Source: CAD feature listing. Evaluate the final solid. Frame: model axes, mm. Face numbers are marked on the shaded views. A direction names the side the tool comes from. Give positions to 0.01 mm unless a question says otherwise; leave off trailing zeros. Loops run counter-clockwise (first coordinate to the right, second up) from the corner with the lowest first, then second, coordinate; pieces in that order, holes last. Notation, with made-up numbers: (10, 51) -> (66, 51) arc R24 ccw to (66, 69) -> close; hole circle Ø4 at (16.25, -12). An arc over 180 degrees is marked (long way). Put each result on its own line as item: value.
```python
from build123d import *

# Parameters (mm, degrees)
BOSS_EXTRUDE1_DEPTH       = 8
CUT_EXTRUDE1_DEPTH        = 46
M2X0_4_TAPPED_HOLE1_D     = 1.6
M2X0_4_TAPPED_HOLE1_DEPTH = 5
M2X0_4_TAPPED_HOLE1_TIP   = 0.480688495


with BuildPart() as part:
    # Sketch1 → Boss-Extrude1 (new body)
    with BuildSketch(Plane.XY):
        Polygon((0, 0), (-8, 0), (-8, -20), (-19, -20), (-19, 25), (-8, 25), align=None)
    extrude(amount=BOSS_EXTRUDE1_DEPTH)

    # Sketch2 → Cut-Extrude1 (cut, through all)
    with BuildSketch(Plane(origin=(0, 25, 0), x_dir=(1, 0, 0), z_dir=(0, 1, 0))):
        Polygon((-19, -4), (-19, -1), (-16, -4), (-19, -7), align=None)
    extrude(amount=-CUT_EXTRUDE1_DEPTH, mode=Mode.SUBTRACT)

    # M2x0.4 Tapped Hole1
    with Locations(Plane(origin=(-8, -6, 4), x_dir=(0, 0, 1), z_dir=(1, 0, 0))):
        with Locations((0, 0), (0, 8)):
            Hole(M2X0_4_TAPPED_HOLE1_D / 2, depth=M2X0_4_TAPPED_HOLE1_DEPTH)
            with Locations((0, 0, -(M2X0_4_TAPPED_HOLE1_DEPTH + M2X0_4_TAPPED_HOLE1_TIP / 2))):  # 118° drill point
                Cone(0, M2X0_4_TAPPED_HOLE1_D / 2, M2X0_4_TAPPED_HOLE1_TIP, mode=Mode.SUBTRACT)


solid = part.part
```
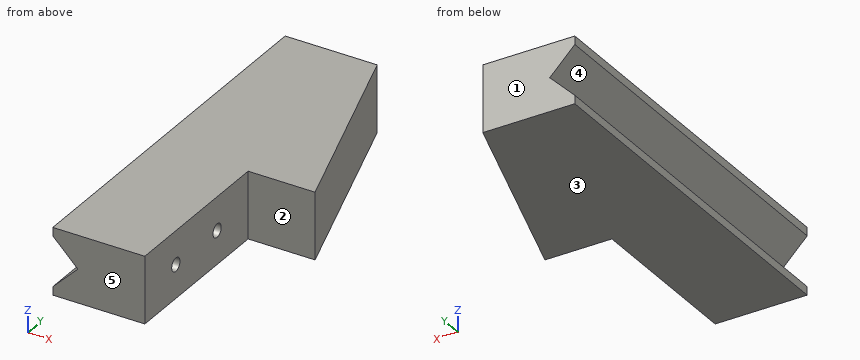
(1) Draft query along Z for the marked faces 3, 4 and 5. Return one class per face: released by +Z, released by -Z, zero draft, split by the parting line, or undercut.
Calculated:
face 3: released by -Z
face 4: undercut
face 5: zero draft
(2) First-contact query: P1, Ø2.5, axis at x = -5, z = 5, coming from the -Y side; P2, Ø1, axis at y = -14, z = 4, coming from the +X side; P3, Ø2, axis at y = -6, z = 4, coming from the +X side. Flat tips, straight axial feed; report the tip coordinate or a pass-through.
Calculated:
P1: stops at y = 0
P2: stops at x = -13.18
P3: stops at x = -8
(3) Reachability of the marked faces 1 and 2 from +Z, -Z, +X, -X, +Y, -Y: full face, straight path, thin tool, end or side. Return the list, or none.
Calculated:
face 1: +Z, -Z, +X, -X, +Y
face 2: +Z, -Z, +X, -Y
(4) Section A-A on x = -16.75. Return loops of the section in (y, z), then the cut area to 4 significant figures.
Calculated:
outline: (-20, 0) -> (25, 0) -> (25, 3.25) -> (-20, 3.25) -> close; (-20, 4.75) -> (25, 4.75) -> (25, 8) -> (-20, 8) -> close
area: 292.5 mm²
(5) Section B-B on y = 18. Return loops of the section in (x, z), then the cut area to 3 significant figures.
Calculated:
outline: (-19, 0) -> (-5.76, 0) -> (-5.76, 8) -> (-19, 8) -> (-19, 7) -> (-16, 4) -> (-19, 1) -> close
area: 96.9 mm²
(6) Section D-D on x = -7. Return loops of the section in (y, z) (3 decimals), then the cut area to 3 significant figures.
Calculated:
outline: (0, 0) -> (21.875, 0) -> (21.875, 8) -> (0, 8) -> close
area: 175 mm²
(7) Section C-C on y = 3. Return loops of the section in (x, z).
Calculated:
outline: (-19, 0) -> (-0.96, 0) -> (-0.96, 8) -> (-19, 8) -> (-19, 7) -> (-16, 4) -> (-19, 1) -> close
(8) Line query: probe 1 along Y at (x, z) = (-9.25, 4); probe 2 along Z at (x, y) = (-11.1, -6); probe 3 along X at (y, z) = (-17.5, 7). Output: solid intervals per line, ascending. Write a range as from..to.
Calculated:
probe 1: y = -20..-14.8, -13.2..-6.8, -5.2..25
probe 2: z = 0..3.2, 4.8..8
probe 3: x = -19..-8
